Build history of the part. All positions in model axes, mm. A direction names the side the tool comes from. Give positions to 0.01 mm unless a question says otherwise; leave off trailing zeros. Order: outer loops, then holes, each group sorted by start corner. A loop starts at its lowest first (then second) coordinate and runs counter-clockwise, first axis right, second up. Notation, with made-up numbers: (-27, 87) - (-22, 87) arc R26 ccw to (-22, 117) - close; hole circle Ø2 at (-28.5, 18.25). An arc over 180 degrees is marked (long way). Write each question's results on one line, items separated by ' | '. Start each with the question number.
1) Cut at C-C on y = -10. List the corners of the cut face in (x, z).
2) Drop flat-ended pins along their axis: pin 1 Ø6 at (x, y) = (-8.5, 5.5) entering from -Z; pin 2 Ø2 at (x, z) = (-12, -14) entering from +Y; pin 3 Ø1.5 at (y, z) = (-5.5, 4) entering from +X; pin 4 Ø1.5 at (x, z) = (11.5, -14.5) entering from -Y. Give the stop position or say it passes through.
3) Drill centre lines: line 1 along Y through (x, z) = (-3, 2); line 2 along Y through (x, z) = (19.5, -7); line 3 along X through (y, z) = (-2.5, 2). Where is each one in solid material? Low to high. Write a range as from..to.
4) Tool access for faces 1 (the face through (-0.163, 7.395, 1.243)), 2 (the face through (0, -13, 0)), 3 (the face through (-2, -12, -4)): list every direction of +Z, -Z, +X, -X, +Y, -Y with a clear straight run to the whole face (end or side of a thin tool).
5) Cut at D-D on y = 5.25. List the corners of the cut face in (x, z), plus the area to 3 significant figures.
from build123d import *

# Parameters (mm, degrees)
F0_R     = 25.1181711361
F0_R_2   = 20.4995111856
F1_DEPTH = 3
F0_R_3   = 15.560509686
F2_DEPTH = 6
F0_R_4   = 10.0770984701
F3_DEPTH = 9
F0_R_5   = 4.2848341216
F4_DEPTH = 12
F0_R_6   = 1.2539122761
F5_DEPTH = 13
F6_DEPTH = 13
F7_DEPTH = 15


# Not quite as in the source:
# - a fillet or chamfer that OpenCascade refuses, or shapes differently, is made with other operations: its cross-section is extruded or revolved along the edge and cut away or added


with BuildPart() as f1:
    # F0 (on Front) → F1 (new body)
    with BuildSketch(Plane.XZ):
        Circle(F0_R)
        Circle(F0_R_2, mode=Mode.SUBTRACT)
    extrude(amount=F1_DEPTH)

    # F0 (on Front) → F2 (join)
    with BuildSketch(Plane.XZ):
        Circle(F0_R_2)
        Circle(F0_R_3, mode=Mode.SUBTRACT)
    extrude(amount=F2_DEPTH)

    # F0 (on Front) → F3 (join)
    with BuildSketch(Plane.XZ):
        Circle(F0_R_3)
        Circle(F0_R_4, mode=Mode.SUBTRACT)
    extrude(amount=F3_DEPTH)

    # F0 (on Front) → F4 (join)
    with BuildSketch(Plane.XZ):
        Circle(F0_R_4)
        Circle(F0_R_5, mode=Mode.SUBTRACT)
    extrude(amount=F4_DEPTH)

    # F0 (on Front) → F5 (join)
    with BuildSketch(Plane.XZ):
        Circle(F0_R_5)
        Circle(F0_R_6, mode=Mode.SUBTRACT)
    extrude(amount=F5_DEPTH)

    # F0 (on Front) → F6 (join)
    with BuildSketch(Plane.XZ):
        Circle(F0_R_6)
    extrude(amount=F6_DEPTH)

    # F0 (on Front) → F7 (join)
    with BuildSketch(Plane.XZ):
        Circle(F0_R_6)
    extrude(amount=-F7_DEPTH)

    # F8: fillet of radius 5 on 4 edges, made by hand

    # F8_s1 → F8_t2 (revolve, cut)
    with BuildSketch(Plane.XY):
        with BuildLine():
            ThreePointArc((25.1181711361, 0), (23.2742082286, -2.1833001327), (20.5355954411, -3))
            Line((20.5355954411, -3), (25.1181711361, -3))
            Line((25.1181711361, -3), (25.1181711361, 0))
        make_face()
    revolve(axis=Axis((0, -3, 0), (0, -1, 0)), mode=Mode.SUBTRACT)

    # F8_s3 → F8_t4 (revolve, cut)
    with BuildSketch(Plane.XY):
        with BuildLine():
            ThreePointArc((20.4995111856, -3), (18.6555482782, -5.1833001327), (15.9169354907, -6))
            Line((15.9169354907, -6), (20.4995111856, -6))
            Line((20.4995111856, -6), (20.4995111856, -3))
        make_face()
    revolve(axis=Axis((0, -6, 0), (0, -1, 0)), mode=Mode.SUBTRACT)

    # F8_s5 → F8_t6 (revolve, cut)
    with BuildSketch(Plane.XY):
        with BuildLine():
            ThreePointArc((15.560509686, -6), (13.7165467785, -8.1833001327), (10.977933991, -9))
            Line((10.977933991, -9), (15.560509686, -9))
            Line((15.560509686, -9), (15.560509686, -6))
        make_face()
    revolve(axis=Axis((0, -9, 0), (0, -1, 0)), mode=Mode.SUBTRACT)

    # F8_s7 → F8_t8 (revolve, cut)
    with BuildSketch(Plane.XY):
        with BuildLine():
            ThreePointArc((10.0770984701, -9), (8.2331355627, -11.1833001327), (5.4945227752, -12))
            Line((5.4945227752, -12), (10.0770984701, -12))
            Line((10.0770984701, -12), (10.0770984701, -9))
        make_face()
    revolve(axis=Axis((0, -12, 0), (0, -1, 0)), mode=Mode.SUBTRACT)


solid = f1.part
Results:
1) outline: circle Ø18.99 at (0, 0)
2) pin 1: through | pin 2: y = 0 | pin 3: x = 18.82 | pin 4: y = -5.65
3) line 1: -13..0 | line 2: -3..0 | line 3: -22.63..22.63
4) face 1: +Y | face 2: +Z, -Z, +X, -X, -Y | face 3: -Y
5) outline: circle Ø2.51 at (0, 0) | area: 4.94 mm^2
